Check sheet for the modelled part. Datum: model origin and axes. Units: mm. A direction names the side the tool comes from. Round coordinates to 2 decimals unless told otherwise and drop trailing zeros. Order: outer loops, then holes, each group sorted by start corner. A loop starts at its lowest first (then second) coordinate and runs counter-clockwise, first axis right, second up. Notation, with made-up numbers: (-27.75, 33) -> (12.25, 33) arc R11 cw to (12.25, 38) -> close; hole circle Ø7 at (-6, 23). An arc over 180 degrees is marked (long way). Answer in a Markdown table with one row per item. Add a question column.
1. Access from +Z, -Z, +X, -X, +Y, -Y to the whole of each face (thin tool, end or side, straight path). Record for faces 5 (the flat face through (15, 57, 17)), 6 (the flat face through (25, 57, 17)), 7 (the flat face through (20, 0, 19)), 8 (the flat face through (30.5, 1, 19)).
2. Sectioned sample at D-D, the plane x = 21. Record the boundary of the cut face in (y, z).
3. Sectioned sample at C-C, the plane z = 15.5. Record the boundary of the cut face in (x, y).
4. Draft check along Z on faces 1 (the flat face through (20.1, 114.6, 17.7)), 2 (the cylindrical face through (5.831, 103.403, 2.465)), 3 (the flat face through (20, -2, 30.5)), 4 (the flat face through (20, 71, 0)). Enter one of: +Z half, -Z half, draft (parallel to the pull), parting line (faces both ways), or undercut.
5. Depth check by flat-ended pin: P1, Ø6, axis at x = 35, y = 105, coming from the -Z side; P2, Ø5, axis at y = -1.5, z = 18.5, coming from the -X side; P3, Ø1, axis at y = 55, z = 29, coming from the -X side; P4, Ø17, axis at x = 21, z = 17, coming from the -Y side. Enter the tip coordinate at first touch or a pass-through.
6. Sectioned sample at B-B, the plane x = 35. Record the boundary of the cut face in (y, z), then the cut area to 3 significant figures.
7. Sectioned sample at A-A, the plane y = 105. Record the boundary of the cut face in (x, z).
8. Material ranges on L1, parallel to X at y = 105, z = 2.4; L2, parallel to Y at x = 35, z = 2; L3, parallel to Y at x = 10.5, z = 8, recorded low to high. Write a range as from..to.
```python
from build123d import *

# Parameters (mm, degrees)
SKETCH_W        = 40
SKETCH_H        = 140
SKETCH_R        = 1.8
PAD_DEPTH       = 5
SKETCH001_W     = 21
SKETCH001_H     = 10
PAD001_DEPTH    = 2
SKETCH002_W     = 21
SKETCH002_H     = 5
PAD002_DEPTH    = 25.5
SKETCH003_W     = 21
SKETCH003_H     = 2
PAD003_DEPTH    = 5
SKETCH004_R     = 1
POCKET_DEPTH    = 100
SKETCH005_W     = 10
SKETCH005_H     = 135
PAD004_DEPTH    = 25
POCKET001_DEPTH = 10


with BuildPart() as part:
    # Sketch → Pad (new body)
    with BuildSketch(Plane.XY):
        with Locations((20, 70)):
            Rectangle(SKETCH_W, SKETCH_H)
        with Locations((5, 135)):
            Circle(SKETCH_R, mode=Mode.SUBTRACT)
        with Locations((35, 135)):
            Circle(SKETCH_R, mode=Mode.SUBTRACT)
        with Locations((5, 105)):
            Circle(SKETCH_R, mode=Mode.SUBTRACT)
        with Locations((35, 105)):
            Circle(SKETCH_R, mode=Mode.SUBTRACT)
    extrude(amount=PAD_DEPTH)

    # Sketch001 (on Face10 of Pad) → Pad001 (join)
    with BuildSketch(Plane.XY.offset(5)):
        with Locations((20, 0)):
            Rectangle(SKETCH001_W, SKETCH001_H)
    extrude(amount=PAD001_DEPTH)

    # Sketch002 (on Face16 of Pad001) → Pad002 (join)
    with BuildSketch(Plane.XY.offset(7)):
        with Locations((20, 2.5)):
            Rectangle(SKETCH002_W, SKETCH002_H)
    extrude(amount=PAD002_DEPTH)

    # Sketch003 (on Face20 of Pad002) → Pad003 (join)
    with BuildSketch(Plane.XZ):
        with Locations((20, 31.5)):
            Rectangle(SKETCH003_W, SKETCH003_H)
    extrude(amount=PAD003_DEPTH)

    # Sketch004 (on Face25 of Pad003) → Pocket (cut)
    with BuildSketch(Plane.XY.offset(32.5)):
        with Locations((11.75, -2)):
            Circle(SKETCH004_R)
        with Locations((28.25, -2)):
            Circle(SKETCH004_R)
    extrude(amount=-POCKET_DEPTH, mode=Mode.SUBTRACT)

    # Sketch005 (on Face5 of Pocket) → Pad004 (join)
    with BuildSketch(Plane.XY.offset(5)):
        with Locations((20, 72.5)):
            Rectangle(SKETCH005_W, SKETCH005_H)
    extrude(amount=PAD004_DEPTH)

    # Sketch006 (on Face16 of Pad004) → Pocket001 (cut)
    with BuildSketch(Plane.YZ.offset(25)):
        Polygon((90, 30), (140, 5), (160, 5), (160, 50), (90, 50), align=None)
    extrude(amount=-POCKET001_DEPTH, mode=Mode.SUBTRACT)


solid = part.part
```
Answer key:
| question | item | result |
|---|---|---|
| 1 | face 5 | +Z, -X, +Y |
| 1 | face 6 | +Z, +X, +Y |
| 1 | face 7 | +X, -X, -Y |
| 1 | face 8 | +Z, +X, +Y, -Y |
| 2 | outline | (-5, 5) -> (0, 5) -> (0, 0) -> (140, 0) -> (140, 5) -> (90, 30) -> (5, 30) -> (5, 32.5) -> (-5, 32.5) -> (-5, 30.5) -> (0, 30.5) -> (0, 7) -> (-5, 7) -> close |
| 3 | outline | (9.5, 0) -> (30.5, 0) -> (30.5, 5) -> (25, 5) -> (25, 119) -> (15, 119) -> (15, 5) -> (9.5, 5) -> close |
| 4 | face 1 | +Z half |
| 4 | face 2 | draft |
| 4 | face 3 | undercut |
| 4 | face 4 | -Z half |
| 5 | P1 | stops at z = 0 |
| 5 | P2 | stops at x = 9.5 |
| 5 | P3 | stops at x = 15 |
| 5 | P4 | stops at y = 0 |
| 6 | outline | (0, 0) -> (103.2, 0) -> (103.2, 5) -> (0, 5) -> close; (106.8, 0) -> (133.2, 0) -> (133.2, 5) -> (106.8, 5) -> close; (136.8, 0) -> (140, 0) -> (140, 5) -> (136.8, 5) -> close |
| 6 | area | 664 mm² |
| 7 | outline | (0, 0) -> (3.2, 0) -> (3.2, 5) -> (0, 5) -> close; (6.8, 0) -> (33.2, 0) -> (33.2, 5) -> (25, 5) -> (25, 22.5) -> (15, 22.5) -> (15, 5) -> (6.8, 5) -> close; (36.8, 0) -> (40, 0) -> (40, 5) -> (36.8, 5) -> close |
| 8 | L1 | x = 0..3.2, 6.8..33.2, 36.8..40 |
| 8 | L2 | y = 0..103.2, 106.8..133.2, 136.8..140 |
| 8 | L3 | y = 0..5 |
